Verification items for this drawing (mm, ordinates from the low corner). A direction names the side the tool comes from. Round coordinates to 2 decimals unless told otherwise and drop trailing zeros. Loops run counter-clockwise (first coordinate to the right, second up) from the corner with the lowest first, then second, coordinate; pieces in that order, holes last. Notation, with made-up numbers: M -32,24.5 L -8,24.5 A19 cw -8,32.5 Z; hole C -9.75,-1 d10. An arc over 180 degrees is marked long. One line per item, written item: value.
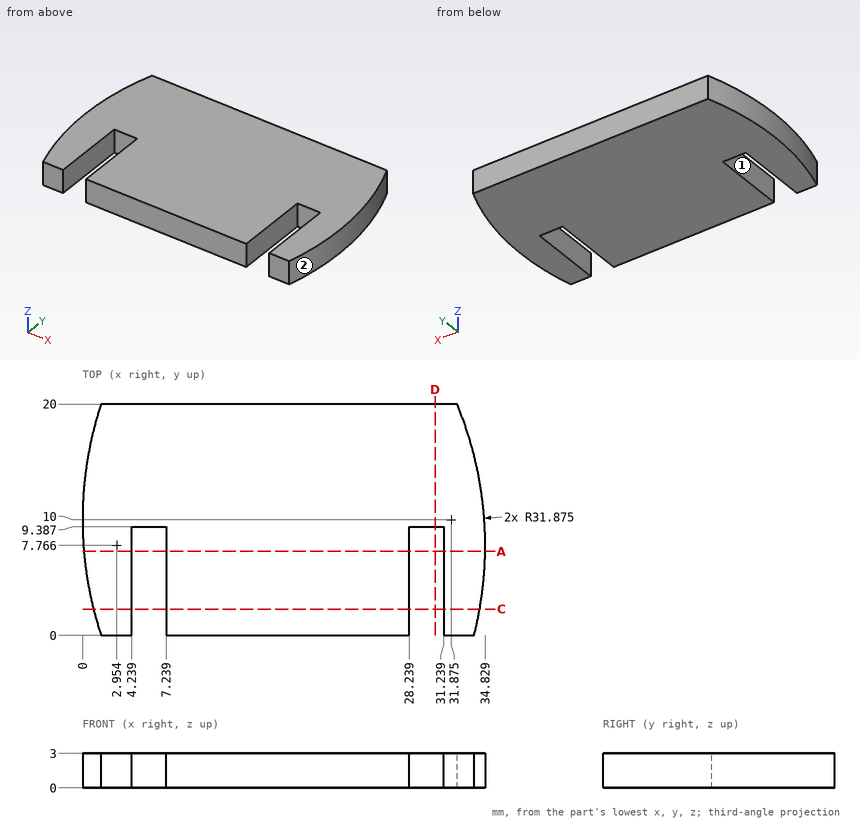
(1) Depth check by flat-ended pin: pin 1 Ø1 at (y, z) = (15, 0.5) entering from -X; pin 2 Ø0.9 at (y, z) = (6, 2) entering from -X; pin 3 Ø1.5 at (x, z) = (29.5, 1.5) entering from -Y. Enter the tip coordinate at first touch or a pass-through.
Completed:
pin 1: stops at x = 0.32
pin 2: stops at x = 0.2
pin 3: stops at y = 9.39
(2) Thickness scan on L1, parallel to X at y = 9.25, z = 1.85 (1 decimal); L2, parallel to X at y = 5.75, z = 2.3 (1 decimal); L3, parallel to Y at x = 29, z = 2.35. Record the ranges inside material, lowest first. Write a range as from..to.
Completed:
L1: x = 0..4.2, 7.2..28.2, 31.2..34.8
L2: x = 0.3..4.2, 7.2..28.2, 31.2..34.8
L3: y = 9.39..20
(3) Sectioned sample at D-D on x = 30.5. Enter the section's corners in (y, z).
Completed:
outline: M 9.39,0 L 20,0 L 20,3 L 9.39,3 Z
(4) Sectioned sample at C-C on y = 2.25. Enter the section's corners in (x, z).
Completed:
outline: M 0.96,0 L 4.24,0 L 4.24,3 L 0.96,3 Z; M 7.24,0 L 28.24,0 L 28.24,3 L 7.24,3 Z; M 31.24,0 L 34.35,0 L 34.35,3 L 31.24,3 Z
(5) Tool access check on the marked faces 1 and 2. Record the directions out of +Z, -Z, +X, -X, +Y, -Y that give a thin tool (end or side, any length) a straight path to the whole face; none if there is none.
Completed:
face 1: +Z, -Z, -Y
face 2: +Z, -Z, +X
(6) Sectioned sample at A-A on y = 7.25. Enter the section's corners in (x, z) (1 decimal).
Completed:
outline: M 0.1,0 L 4.2,0 L 4.2,3 L 0.1,3 Z; M 7.2,0 L 28.2,0 L 28.2,3 L 7.2,3 Z; M 31.2,0 L 34.8,0 L 34.8,3 L 31.2,3 Z
